from build123d import *

# Parameters (mm, degrees)
F1_W     = 35
F1_H     = 100
F2_DEPTH = 1.2
F1_W_2   = 37.4
F1_H_2   = 102.4
F3_DEPTH = 2.4
F4_R     = 2
F5_W     = 1.5
F5_H     = 79.3849229813
F6_DEPTH = 1.2
F7_R     = 5


with BuildPart() as f2:
    # F1 (on Top) → F2 (new body)
    with BuildSketch(Plane.XY):
        Rectangle(F1_W, F1_H)
    extrude(amount=F2_DEPTH)

    # F1 (on Top) → F3 (join)
    with BuildSketch(Plane.XY):
        Rectangle(F1_W_2, F1_H_2)
        Rectangle(F1_W, F1_H, mode=Mode.SUBTRACT)
    extrude(amount=F3_DEPTH)

    # F4
    f4_edges = [f2.edges().sort_by_distance(p)[0] for p in [
        (-18.7, -51.2, 1.2),
        (18.7, -51.2, 1.2),
        (18.7, 51.2, 1.2),
        (-18.7, 51.2, 1.2),
    ]]
    fillet(f4_edges, radius=F4_R)

    # F5 (on face) → F6 (join)
    with BuildSketch(Plane.XY):
        Polygon((-23.8, -43.636681512), (-18.7, -43.636681512), (-18.7, 43.636681512), (-23.8, 43.636681512), (-23.8, 0), align=None)
        with Locations((-21.25, 0)):
            Rectangle(F5_W, F5_H, mode=Mode.SUBTRACT)
        Polygon((23.8, -43.636681512), (23.8, 0), (23.8, 43.636681512), (18.7, 43.636681512), (18.7, -43.636681512), align=None)
        with Locations((21.25, 0)):
            Rectangle(F5_W, F5_H, mode=Mode.SUBTRACT)
    extrude(amount=F6_DEPTH)

    # F7
    f7_edges = [f2.edges().sort_by_distance(p)[0] for p in [
        (-23.8, 43.636682, 0.6),
        (23.8, 43.636682, 0.6),
        (23.8, -43.636682, 0.6),
        (-23.8, -43.636682, 0.6),
    ]]
    fillet(f7_edges, radius=F7_R)


solid = f2.part
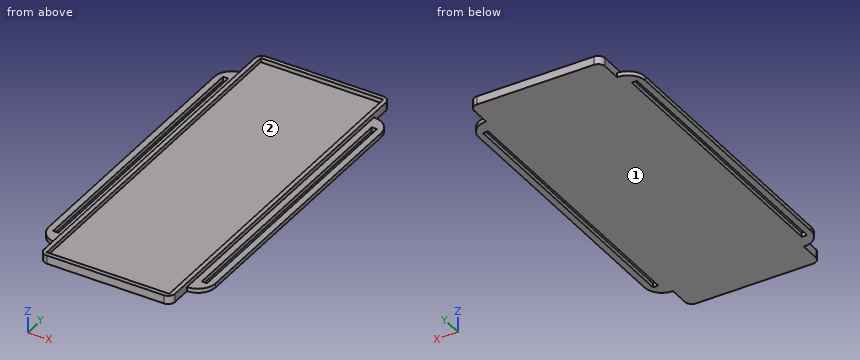
CAD build for the part. Positions are in the model's coordinates, mm. Face numbers are marked on the shaded views. Round coordinates to 2 decimals unless told otherwise and drop trailing zeros. Loops run counter-clockwise (first coordinate to the right, second up) from the corner with the lowest first, then second, coordinate; pieces in that order, holes last.
(1) Drop flat-ended pins along their axis: pin 1 (0.6 mm diameter, centred on x = 21, z = 1, fed in from +Y); pin 2 (1.3 mm diameter, centred on x = 21, z = 0.5, fed in from -Y); pin 3 (1.5 mm diameter, centred on x = -20.5, y = -12, fed in from +Z). Give the stop position or say it passes through.
(2) Cut at A-A (y = 6). Give the cut face in (x, z), plus the area to 3 significant figures.
(3) Cut at B-B (z = 0.4). Give the cut face in (x, y).
(4) Wall check: line 1 along X through (y, z) = (-21.5, 2.15); line 2 along Y through (x, z) = (-12.5, 1.75); line 3 along X through (y, z) = (-4.5, 0.85). Give the ranges that are in metal, low to high.
(5) Cut at C-C (x = -6.5). Give the cut face in (y, z), plus the area to 3 significant figures.
(6) Two-plate mould, pull along Y, no slides. Class the marked faces 1 and 2: +Y half, -Y half, draft (parallel to the pull), parting line (faces both ways), or undercut.
Findings below:
1. pin 1: stops at y = 43.26
1. pin 2: stops at y = -43.39
1. pin 3: stops at z = 1.2
2. outline: (-23.8, 0) - (-22, 0) - (-22, 1.2) - (-23.8, 1.2) - close; (-20.5, 0) - (20.5, 0) - (20.5, 1.2) - (18.7, 1.2) - (18.7, 2.4) - (17.5, 2.4) - (17.5, 1.2) - (-17.5, 1.2) - (-17.5, 2.4) - (-18.7, 2.4) - (-18.7, 1.2) - (-20.5, 1.2) - close; (22, 0) - (23.8, 0) - (23.8, 1.2) - (22, 1.2) - close
2. area: 56.4 mm2
3. outline: (-23.8, -38.64) arc R5 ccw to (-18.8, -43.64) - (-18.7, -43.64) - (-18.7, -49.2) arc R2 ccw to (-16.7, -51.2) - (16.7, -51.2) arc R2 ccw to (18.7, -49.2) - (18.7, -43.64) - (18.8, -43.64) arc R5 ccw to (23.8, -38.64) - (23.8, 38.64) arc R5 ccw to (18.8, 43.64) - (18.7, 43.64) - (18.7, 49.2) arc R2 ccw to (16.7, 51.2) - (-16.7, 51.2) arc R2 ccw to (-18.7, 49.2) - (-18.7, 43.64) - (-18.8, 43.64) arc R5 ccw to (-23.8, 38.64) - close; hole (-22, -39.69) - (-20.5, -39.69) - (-20.5, 39.69) - (-22, 39.69) - close; hole (20.5, -39.69) - (22, -39.69) - (22, 39.69) - (20.5, 39.69) - close
4. line 1: x = -18.7 to -17.5, 17.5 to 18.7
4. line 2: y = -51.2 to -50, 50 to 51.2
4. line 3: x = -23.8 to -22, -20.5 to 20.5, 22 to 23.8
5. outline: (-51.2, 0) - (51.2, 0) - (51.2, 2.4) - (50, 2.4) - (50, 1.2) - (-50, 1.2) - (-50, 2.4) - (-51.2, 2.4) - close
5. area: 126 mm2
6. face 1: draft
6. face 2: undercut
